Build history of the part. All positions in model axes, mm. A direction names the side the tool comes from. Give positions to 0.01 mm unless a question says otherwise; leave off trailing zeros. Write each loop counter-clockwise with the first axis right and the second up, starting at its lowest first coordinate (ties: lowest second). Pieces come first, ordered by that corner, then holes. Notation, with made-up numbers: M 48,-9.75 L 72,-9.75 A11 ccw 72,4.25 Z; hole C 29,-26 d2. An arc over 180 degrees is marked long. Return JSON: item names as keys, results as strings. Group by question number.
Q1. Band-saw the part on C-C, the plane y = 22.5. Give the cut face in (x, z), then the cut area to 3 significant figures.
Q2. Wall check: probe 1 along Y at (x, z) = (29.5, -94.5); probe 2 along X at (y, z) = (25.5, 35.5); probe 3 along X at (y, z) = (59, -105). Give the ranges that are in metal, low to high.
Q3. Flat gauge pins, fed straight in: pin 1 Ø1 at (y, z) = (15, -5) entering from -X; pin 2 Ø6 at (x, z) = (-4, -1) entering from +Y; pin 3 Ø12 at (x, y) = (114.5, 47) entering from -Z. Where does each tip first touch, or does it go through?
Q4. Tool access for faces 1 (the cylindrical face through (27.624, 69.02, -125.097)), 2 (the cylindrical face through (-12, 39, 25)), 3 (the flat face through (0, 2, 25)): list every direction of +Z, -Z, +X, -X, +Y, -Y with a clear straight run to the whole face (end or side of a thin tool).
Q5. Band-saw the part on B-B, the plane y = 109.5. Give the cut face in (x, z), then the cut area to 3 significant figures.
from build123d import *

# Parameters (mm, degrees)
BOTTOM_LEVEL_DEPTH = 5
MID_LEVEL_DEPTH    = 35
GUARD_RAIL_DEPTH   = 100
ROUNDING_R         = 5


with BuildPart() as part:
    # Sketch1 → Bottom level (new body)
    with BuildSketch(Plane(origin=(0, 0, 0), x_dir=(1, 0, 0), z_dir=(0, 1, 0))):
        with BuildLine():
            Line((150, 150), (150, 175))
            ThreePointArc((150, 175), (26.256313292, 123.743686708), (-25, 0))
            Line((-25, 0), (-25, -50))
            Line((-25, -50), (0, -50))
            Line((0, -50), (0, 0))
            ThreePointArc((0, 0), (43.933982822, 106.066017178), (150, 150))
        make_face()
    extrude(amount=BOTTOM_LEVEL_DEPTH)

    # Sketch2 → Mid level (add)
    with BuildSketch(Plane(origin=(0, 5, 0), x_dir=(1, 0, 0), z_dir=(0, 1, 0))):
        with BuildLine():
            Line((-25, 0), (-25, -50))
            Line((-25, -50), (-10, -50))
            Line((-10, -50), (-10, 0))
            ThreePointArc((-10, 0), (36.86291501, 113.13708499), (150, 160))
            Line((150, 160), (150, 175))
            ThreePointArc((150, 175), (26.256313292, 123.743686708), (-25, 0))
        make_face()
    extrude(amount=MID_LEVEL_DEPTH)

    # Sketch3 → Guard rail (add)
    with BuildSketch(Plane(origin=(0, 40, 0), x_dir=(1, 0, 0), z_dir=(0, 1, 0))):
        with BuildLine():
            Line((-25, 0), (-25, -50))
            Line((-25, -50), (-20, -50))
            Line((-20, -50), (-20, 0))
            ThreePointArc((-20, 0), (29.791847198, 120.208152802), (150, 170))
            Line((150, 170), (150, 175))
            ThreePointArc((150, 175), (26.256313292, 123.743686708), (-25, 0))
        make_face()
    extrude(amount=GUARD_RAIL_DEPTH)

    # Rounding
    rounding_edges = [part.edges().sort_by_distance(p)[0] for p in [
        (-10, 5, 25),
        (-10, 40, 25),
        (-20, 40, 25),
        (36.86291501, 5, -113.13708499),
        (36.86291501, 40, -113.13708499),
        (29.791847198, 40, -120.208152802),
    ]]
    fillet(rounding_edges, radius=ROUNDING_R - 0.0001)  # a hair under: the kernel refuses the full size


solid = part.part
From the geometry:
{
 "1": {"outline": "M -25,0 A175 ccw 150,-175 L 150,-160 A160 cw -10,0 L -10,50 L -25,50 Z", "area": "4,700 mm^2"},
 "2": {"probe 1": "y = 0 to 5", "probe 2": "x = -25 to -10", "probe 3": "x = 10 to 16.3"},
 "3": {"pin 1": "stops at x = -24.94", "pin 2": "stops at y = 5.42", "pin 3": "stops at z = -172.5"},
 "4": {"face 1": "-Z, -X, +Y, -Y", "face 2": "+Z, +X, +Y", "face 3": "+Z, +X, +Y, -Y"},
 "5": {"outline": "M -25,0 A175 ccw 150,-175 L 150,-170 A170 cw -20,0 L -20,50 L -25,50 Z", "area": "1,600 mm^2"}
}
